Autodesk Inventor part; units mm, degrees
ref_plane "YZ Plane" through (0, 0, 0) normal (1, 0, 0) x (0, 1, 0)
ref_plane "XZ Plane" through (0, 0, 0) normal (0, 1, 0) x (-1, 0, 0)
ref_plane "XY Plane" through (0, 0, 0) normal (0, 0, 1) x (1, 0, 0)
sketch "Sketch1" plane through (0, 0, 0) normal (0, 1, 0) x (-1, 0, 0)
  circle A0 centre (0, 0) radius 27.5
  point P0 (20, 0)
  point P1 (14.1421, 14.1421)
  point P2 (0, 20)
  point P3 (-14.1421, 14.1421)
  point P4 (-20, 0)
  point P5 (-14.1421, -14.1421)
  point P6 (0, -20)
  point P7 (14.1421, -14.1421)
  dimension "d0" = 55
  dimension "d19" = 20
  dimension "d22" = 360
extrude "Extrusion1" add sketch "Sketch1" against normal blind 28
sketch "Sketch2" plane through (0, -28, 0) normal (0, -1, 0) x (1, 0, 0)
  circle A0 centre (0, 0) radius 27.5
  line L0 (0, 27.5) -> (45, 27.5)
  line L1 (45, 27.5) -> (45, -27.5)
  line L2 (45, -27.5) -> (0, -27.5)
  dimension "d15" = 45
  dimension "d16" = 55
extrude "Extrusion2" add sketch "Sketch2" against normal blind 27 contours A0 L0 L1 L2
hole "Hole1" at (0, 0, 20) at (0, 0, -20) direction (0, -1, 0) diameter 6 depth 3 tip angle 118
hole "Hole2" at (-14.1421, 0, 14.1421) at (14.1421, 0, 14.1421) at (14.1421, 0, -14.1421) at (-14.1421, 0, -14.1421) direction (0, -1, 0) diameter 4.917 depth 8 tip angle 118
sketch "Sketch3" plane through (0, -28, 0) normal (0, -1, 0) x (1, 0, 0)
  arc A0 (0, 27.5) -> (0, -27.5) centre (0, 0) ccw
  circle A1 centre (0, 0) radius 12.5
  circle A2 centre (0, 0) radius 20
  circle A3 centre (20, 0) radius 3
  circle A4 centre (14.1421, 14.1421) radius 3
  circle A5 centre (0, 20) radius 3
  circle A6 centre (-14.1421, 14.1421) radius 3
  circle A7 centre (-20, 0) radius 3
  circle A8 centre (-14.1421, -14.1421) radius 3
  circle A9 centre (0, -20) radius 3
  circle A10 centre (14.1421, -14.1421) radius 3
  dimension "d44" = 40
  dimension "d38" = 25
  dimension "d45" = 6
  dimension "d48" = 360
extrude "Extrusion3" add sketch "Sketch3" along normal blind 3 contours A1
chamfer "Chamfer1" distance 0.5 angle 45 1 edges at (-12.5, -31, 0)
extrude "Extrusion4" add sketch "Sketch3" along normal blind 6 contours A4 A2 | A2 A4 | A10 A2 | A2 A10 | A6 A2 | A2 A6 | A8 A2 | A2 A8
thread "Thread1"
thread "Thread2"
thread "Thread3"
thread "Thread4"
chamfer "Chamfer2" distance 0.5 angle 45 1 edges at (-17.1421, -34, -14.1421)
chamfer "Chamfer3" distance 0.5 angle 45 1 edges at (-17.1421, -34, 14.1421)
chamfer "Chamfer4" distance 0.5 angle 45 1 edges at (11.1421, -34, 14.1421)
chamfer "Chamfer5" distance 0.5 angle 45 1 edges at (11.1421, -34, -14.1421)
hole "Hole3" at (0, -28, 20) at (0, -28, -20) direction (0, 1, 0) diameter 6 depth 3 tip angle 118
properties part number "CFS055CA501U"
Read the model definition and answer for the solid it produces. Units are mm, in the model's axes. A direction names the side the tool comes from. Coordinates: 2 decimals unless noted, no trailing zeros. Order: outer loops, then holes, each group sorted by start corner. A loop starts at its lowest first (then second) coordinate and runs counter-clockwise, first axis right, second up. Notation, with made-up numbers: (-4, 67.25) - (16, 67.25) arc R26 cw to (16, 100.25) - close; hole circle Ø11 at (-35.5, -10.75). An arc over 180 degrees is marked (long way). Use one line per item in the form item = value.
(1) For a pull along Z with two mould halves and no side action, classify faces 3 (the face through (-26.23, -13.8, 8.26)), 4 (the face through (0, -26, 23)) as pulls with the +Z half, pulls with the -Z half, needs draft (parallel to the pull), parting line crosses it, or undercut.
Computed values:
face_3 = parting line crosses it
face_4 = undercut
(2) Section C-C, the plane x = 33.5 is taken. Give the vertices of the cut face in (y, z), then the cut area to 4 significant figures.
Computed values:
outline = (-28, -27.5) - (-1, -27.5) - (-1, 27.5) - (-28, 27.5) - close
area = 1,485 mm²
(3) Which of the six approach directions +Z, -Z, +X, -X, +Y, -Y give full straight-line access (tool end or side, diameter ignored) to faces 1 (the face through (11.93, -30.71, -16.17)), 2 (the face through (0, -2, -23))?
Computed values:
face_1 = -Y
face_2 = +Y
(4) Given pin 1 Ø7 at (x, z) = (0, 20) entering from -Y; pin 2 Ø8 at (x, y) = (-6.5, -17) entering from +Z; pin 3 Ø6 at (y, z) = (-11, 12.5) entering from -X, each flat-ended and moving along its own axis, determine where each tip first touches the part or whether it passes through.
Computed values:
pin_1 = -28
pin_2 = 27.39
pin_3 = -25.81
(5) Straight lines are drawn through the part: L1, parallel to Z at x = 0, y = -25.8; L2, parallel to Y at x = 22, z = -3.5; L3, parallel to Z at x = -1, y = -16. For each, find the intervals that lie inside material, in ascending order.
Computed values:
L1 = -27.5 to -23, -17 to 17, 23 to 27.5
L2 = -28 to 0
L3 = -27.48 to 27.48
(6) Section B-B, the plane y = -13 is taken. Give the vertices of the cut face in (x, z).
Computed values:
outline = (0, -27.5) - (45, -27.5) - (45, 27.5) - (0, 27.5) arc R27.5 ccw to start
(7) Section A-A, the plane z = 0 is taken. Give the vertices of the cut face in (x, y), then the cut area to 3 significant figures.
Computed values:
outline = (-27.5, -28) - (-12.5, -28) - (-12.5, -30.5) - (-12, -31) - (12, -31) - (12.5, -30.5) - (12.5, -28) - (45, -28) - (45, -1) - (27.5, -1) - (27.5, 0) - (-27.5, 0) - close
area = 2,090 mm²
